For this review, take the finished solid that the model builds, in its own axes (mm). A direction names the side the tool comes from. Coordinates: 2 decimals unless noted, no trailing zeros. Loops run counter-clockwise (first coordinate to the right, second up) from the corner with the lowest first, then second, coordinate; pieces in that order, holes last. Notation, with made-up numbers: M 79.25,61 L 113.25,61 A5 ccw 113.25,69 Z; hole C -4,53.25 d9. An arc over 180 degrees is marked long. Use one line per item in the form item = value.
```python
from build123d import *

# Parameters (mm, degrees)
F0_W     = 60
F0_H     = 50
F1_DEPTH = 20
F2_W     = 40
F2_H     = 50
F3_DEPTH = 40
F5_DEPTH = 10
F7_DEPTH = 40


with BuildPart() as f1:
    # F0 (on Top) → F1 (new body)
    with BuildSketch(Plane.XY):
        with Locations((30, 25)):
            Rectangle(F0_W, F0_H)
    extrude(amount=F1_DEPTH)

    # F2 (on face) → F3 (join)
    with BuildSketch(Plane.XY.offset(20)):
        with Locations((30, 25)):
            Rectangle(F2_W, F2_H)
    extrude(amount=F3_DEPTH)

    # F4 (on face) → F5 (cut)
    with BuildSketch(Plane(origin=(0, 0, 0), x_dir=(1, 0, 0), z_dir=(0, 0, -1))):
        Polygon((30, 0), (0, 0), (30, -50), (60, -50), align=None)
    extrude(amount=-F5_DEPTH, mode=Mode.SUBTRACT)

    # F6 (on face) → F7 (cut)
    with BuildSketch(Plane.XY.offset(60)):
        Polygon((20, 50), (10, 50), (10, 40), align=None)
    extrude(amount=-F7_DEPTH, mode=Mode.SUBTRACT)

    # F12: sweep along a path in F11
    with BuildLine(Plane(origin=(30, 0, 0), x_dir=(0, -1, 0), z_dir=(-1, 0, 0))) as f12_path:
        Line((0, 45), (-50, 60))
    # F8 (on face) → F12 (sweep, cut)
    with BuildSketch(Plane.XY.offset(60)):
        Polygon((30, 50), (10, 0), (30, 0), align=None)
        Polygon((30, 50), (30, 0), (50, 0), align=None)
    sweep(path=f12_path.line, mode=Mode.SUBTRACT)


solid = f1.part
```
1. Wall thickness on line 1 along X through (y, z) = (17.5, 30); line 2 along Z through (x, y) = (11, 41.5); line 3 along X through (y, z) = (13, 52): over which ranges is each line inside the solid? List them lowest first. Write a range as from..to.
Computed values:
line_1 = 10..50
line_2 = 0..20
line_3 = 10..25.87, 34.13..50
2. Consider section B-B on z = 7. Write out the cut boundary in (x, y).
Computed values:
outline = M 0,0 L 30,50 L 0,50 Z; M 30,0 L 60,0 L 60,50 Z
3. Tool access review of faces 1 (the face through (24.502, 17.161, 54.272)), 2 (the face through (15, 25, 5)), 3 (the face through (50, 25, 40)), 4 (the face through (10, 20, 40)): name each direction out of +Z, -Z, +X, -X, +Y, -Y from which nothing blocks a thin tool from reaching the whole face with its end or side.
Computed values:
face_1 = +Z, -Y
face_2 = -Z, -Y
face_3 = +Z, +X, +Y, -Y
face_4 = +Z, -X, +Y, -Y
4. Consider section C-C on y = 29.5. Write out the cut boundary in (x, z), plus the area to 3 significant figures.
Computed values:
outline = M 0,0 L 17.7,0 L 17.7,10 L 47.7,10 L 47.7,0 L 60,0 L 60,20 L 50,20 L 50,60 L 38.2,60 L 30,53.85 L 21.8,60 L 10,60 L 10,20 L 0,20 Z
area = 2,450 mm2
5. Consider section A-A on x = 42. Write out the cut boundary in (y, z), plus the area to 3 significant figures.
Computed values:
outline = M 0,0 L 20,0 L 20,10 L 50,10 L 50,60 L 20,60 L 0,54 Z
area = 2,640 mm2
6. For pin 1 Ø20 at (y, z) = (20.5, 33.5) entering from +X; pin 2 Ø11 at (x, y) = (57, 25.5) entering from +Z; pin 3 Ø20 at (y, z) = (19.5, 40.5) entering from -X, all flat-tipped, find the tip position at first contact; note any pin that passes through.
Computed values:
pin_1 = 50
pin_2 = 20
pin_3 = 10
7. Consider section D-D on z = 37. Write out the cut boundary in (x, y), plus the area to 3 significant figures.
Computed values:
outline = M 10,0 L 50,0 L 50,50 L 20,50 L 10,40 Z
area = 1,950 mm2
